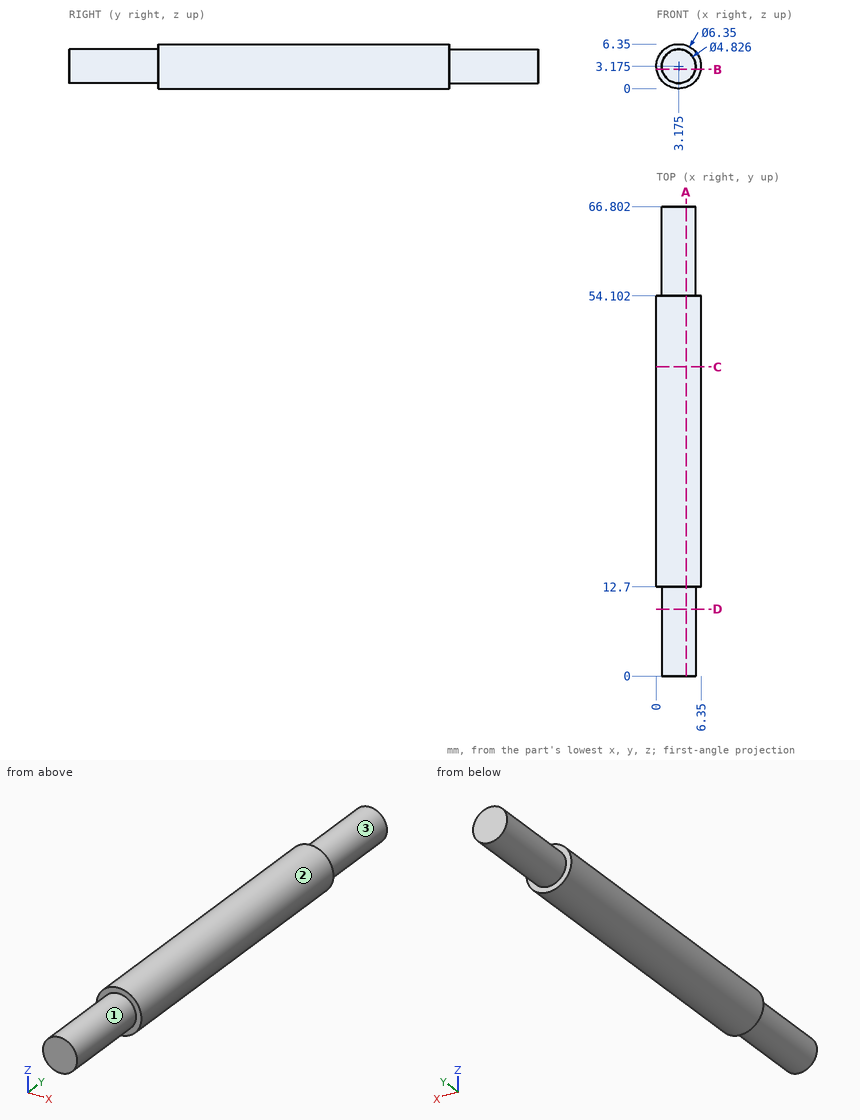
Drawing for the job (mm, zero at the part's lowest x, y, z). A direction names the side the tool comes from. Round coordinates to 2 decimals unless told otherwise and drop trailing zeros. Order: outer loops, then holes, each group sorted by start corner. A loop starts at its lowest first (then second) coordinate and runs counter-clockwise, first axis right, second up.
Item 1: Saw through at C-C on y = 44. Write the cut outline in (x, z) (3 decimals), then the cut area to 3 significant figures.
Item 2: Saw through at D-D on y = 9.5. Write the cut outline in (x, z) (3 decimals).
Item 3: Saw through at B-B on z = 2.75. Write the cut outline in (x, y).
Item 4: Tool access for the marked faces 1, 2 and 3: list every direction of +Z, -Z, +X, -X, +Y, -Y with a clear straight run to the whole face (end or side of a thin tool).
Item 5: Probe line 1 along Y through (x, z) = (1, 5.25); line 2 along X through (y, z) = (26, 3); line 3 along Z through (x, y) = (3, 8). List the from-to ranges inside material, lowest first.
Item 6: Saw through at A-A on x = 4.25. Write the cut outline in (y, z), then the cut area to 3 significant figures.
Reported:
1. outline: circle Ø6.35 at (3.175, 3.175)
1. area: 31.7 mm2
2. outline: circle Ø4.826 at (3.175, 3.175)
3. outline: (0.03, 12.7) - (0.8, 12.7) - (0.8, 0) - (5.55, 0) - (5.55, 12.7) - (6.32, 12.7) - (6.32, 54.1) - (5.55, 54.1) - (5.55, 66.8) - (0.8, 66.8) - (0.8, 54.1) - (0.03, 54.1) - close
4. face 1: -Y
4. face 2: +Y, -Y
4. face 3: +Y
5. line 1: y = 12.7 to 54.1
5. line 2: x = 0 to 6.35
5. line 3: z = 0.77 to 5.58
6. outline: (0, 1.01) - (12.7, 1.01) - (12.7, 0.19) - (54.1, 0.19) - (54.1, 1.01) - (66.8, 1.01) - (66.8, 5.34) - (54.1, 5.34) - (54.1, 6.16) - (12.7, 6.16) - (12.7, 5.34) - (0, 5.34) - close
6. area: 357 mm2
